The model under review builds one solid part; all positions refer to its coordinate system, in mm. Round coordinates to 2 decimals unless told otherwise and drop trailing zeros. Write each loop counter-clockwise with the first axis right and the second up, starting at its lowest first coordinate (ties: lowest second). Pieces come first, ordered by that corner, then holes. Notation, with made-up numbers: (-33, 17.5) - (26, 17.5) arc R32 cw to (26, 48.5) - close; hole circle Ø7 at (13.5, 80.5). An arc over 180 degrees is marked (long way). Use one line per item in the form item = value.
from build123d import *

# Parameters (mm, degrees)
F0_W     = 20
F0_H     = 10
F0_W_2   = 18.5
F0_H_2   = 11
F1_DEPTH = 6


with BuildPart() as f1:
    # F0 (on Right) → F1 (new body)
    with BuildSketch(Plane.YZ):
        Polygon((-60.931503, 42.813338), (-54.931503, 42.813338), (-54.931503, -33.186662), (-60.931503, -33.186662), (-60.931503, -43.186662), (-54.931503, -43.186662), (-54.931503, -69.186662), (-49.931503, -69.186662), (-49.931503, -63.186662), (-39.931503, -63.186662), (-39.931503, -69.186662), (-29.931503, -69.186662), (-29.931503, -63.186662), (-19.931503, -63.186662), (-19.931503, -69.186662), (-14.931503, -69.186662), (-14.931503, -43.186662), (-8.931503, -43.186662), (-8.931503, -33.186662), (-14.931503, -33.186662), (-14.931503, 42.813338), (-8.931503, 42.813338), (-8.931503, 52.813338), (-14.931503, 52.813338), (-14.931503, 78.813338), (-19.931503, 78.813338), (-19.931503, 72.813338), (-29.931503, 72.813338), (-29.931503, 78.813338), (-39.931503, 78.813338), (-39.931503, 72.813338), (-49.931503, 72.813338), (-49.931503, 78.813338), (-54.931503, 78.813338), (-54.931503, 52.813338), (-60.931503, 52.813338), align=None)
        with Locations((-30.681503, -51.186662)):
            Rectangle(F0_W, F0_H, mode=Mode.SUBTRACT)
        with Locations((-29.931503, 5.313338)):
            Rectangle(F0_W_2, F0_H_2, mode=Mode.SUBTRACT)
        with Locations((-29.931503, 21.313338)):
            Rectangle(F0_W_2, F0_H_2, mode=Mode.SUBTRACT)
        with Locations((-29.931503, 37.313338)):
            Rectangle(F0_W_2, F0_H_2, mode=Mode.SUBTRACT)
    extrude(amount=F1_DEPTH)


solid = f1.part
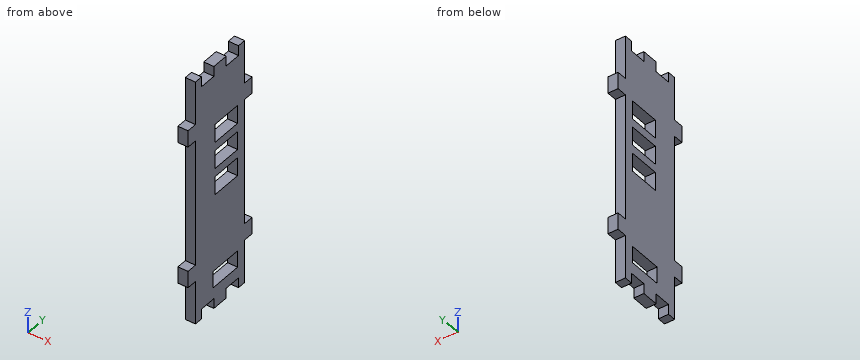
(1) To check wall thickness, follow L1, parallel to Z at x = 5.85, y = -21; L2, parallel to Z at x = 5.5, y = -11; L3, parallel to Z at x = 4.4, y = -40. State the ranges of each line that lie inside material, in increasing order.
Geometry results:
L1 = -63.19 to -56.19, -46.19 to -0.19, 10.81 to 15.81, 26.81 to 31.81, 42.81 to 72.81
L2 = -43.19 to -33.19, 42.81 to 52.81
L3 = -63.19 to -56.19, -46.19 to 72.81
(2) Add section D-D on x = 3.85. Count the separate pieces of the cut face and the enclosed holes in it, then the cut area to 3 significant figures.
Geometry results:
separate_pieces = 1
enclosed_holes = 4
area = 5,110 mm2
(3) Add section B-B on z = -54. Write out the cut boundary in (x, y), then the cut area to 3 significant figures.
Geometry results:
outline = (0, -54.93) - (6, -54.93) - (6, -40.68) - (0, -40.68) - close; (0, -20.68) - (6, -20.68) - (6, -14.93) - (0, -14.93) - close
area = 120 mm2
(4) Add section A-A on y = -27. Write out the cut boundary in (x, z), then the cut area to 3 significant figures.
Geometry results:
outline = (0, -63.19) - (6, -63.19) - (6, -56.19) - (0, -56.19) - close; (0, -46.19) - (6, -46.19) - (6, -0.19) - (0, -0.19) - close; (0, 10.81) - (6, 10.81) - (6, 15.81) - (0, 15.81) - close; (0, 26.81) - (6, 26.81) - (6, 31.81) - (0, 31.81) - close; (0, 42.81) - (6, 42.81) - (6, 72.81) - (0, 72.81) - close
area = 558 mm2
(5) Insertion check: P1, Ø1.8, axis at x = 3, z = 75.5, coming from the +Y side; P2, Ø1.8, axis at x = 2, y = -13.5, coming from the +Z side; P3, Ø3, axis at x = 2.5, y = -29, coming from the +Z side; P4, Ø1.5, axis at x = 4.5, z = 13.5, coming from the -Y side. Each pin has a flat end and moves straight along its axis. Give the tip position at first contact, or say it passes through.
Geometry results:
P1 = -14.93
P2 = 52.81
P3 = 78.81
P4 = -54.93
(6) Add section C-C on y = -35. Write out the cut boundary in (x, z), then the cut area to 3 significant figures.
Geometry results:
outline = (0, -69.19) - (6, -69.19) - (6, -56.19) - (0, -56.19) - close; (0, -46.19) - (6, -46.19) - (6, -0.19) - (0, -0.19) - close; (0, 10.81) - (6, 10.81) - (6, 15.81) - (0, 15.81) - close; (0, 26.81) - (6, 26.81) - (6, 31.81) - (0, 31.81) - close; (0, 42.81) - (6, 42.81) - (6, 78.81) - (0, 78.81) - close
area = 630 mm2
